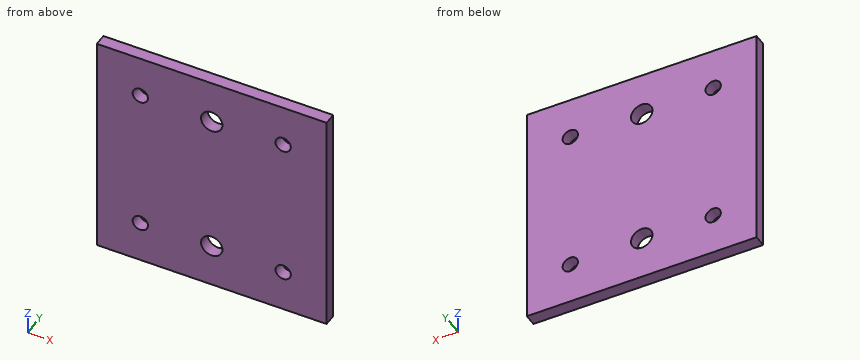
```python
from build123d import *

# Parameters (mm, degrees)
SKETCH1_W           = 150
SKETCH1_H           = 7.962213225
BOSS_EXTRUDE1_DEPTH = 150
SKETCH2_R           = 7
CUT_EXTRUDE1_DEPTH  = 8.962213225
SKETCH3_R           = 5
CUT_EXTRUDE2_DEPTH  = 8.962213225


with BuildPart() as part:
    # Sketch1 → Boss-Extrude1 (new body)
    with BuildSketch(Plane(origin=(0, 0, 0), x_dir=(0, 0, -1), z_dir=(1, 0, 0))):
        with Locations((75, -3.981106613)):
            Rectangle(SKETCH1_W, SKETCH1_H)
    extrude(amount=BOSS_EXTRUDE1_DEPTH)

    # Sketch2 → Cut-Extrude1 (cut, through all)
    with BuildSketch(Plane(origin=(0, 0, 0), x_dir=(1, 0, 0), z_dir=(0, 1, 0))):
        with Locations((74.999907539, 121.3473939)):
            Circle(SKETCH2_R)
        with Locations((74.999907539, 28.6526061)):
            Circle(SKETCH2_R)
    extrude(amount=-CUT_EXTRUDE1_DEPTH, mode=Mode.SUBTRACT)

    # Sketch3 → Cut-Extrude2 (cut, through all)
    with BuildSketch(Plane.XZ.offset(7.962213225)):
        with Locations((28.371496461, -122.5)):
            Circle(SKETCH3_R)
        with Locations((28.371496461, -27.5)):
            Circle(SKETCH3_R)
        with Locations((121.628503539, -27.5)):
            Circle(SKETCH3_R)
        with Locations((121.628503539, -122.5)):
            Circle(SKETCH3_R)
    extrude(amount=-CUT_EXTRUDE2_DEPTH, mode=Mode.SUBTRACT)


solid = part.part
```
Source: CAD feature listing. Evaluate the final solid. Frame: model axes, mm. Give positions to 0.01 mm unless a question says otherwise; leave off trailing zeros. Loops run counter-clockwise (first coordinate to the right, second up) from the corner with the lowest first, then second, coordinate; pieces in that order, holes last. Notation, with made-up numbers: (67.25, 60) -> (87.25, 60) arc R31 ccw to (87.25, 96) -> close; hole circle Ø9 at (78, 43). An arc over 180 degrees is marked (long way). Use a Markdown table: item, result. Add a question column.
(1) Section query B-B (y = -6.25). Output: boundary loops of the cut face in (x, z).
(2) Ray query, line 1 (X direction, y = -3.5, z = -25.5); line 2 (Z direction, x = 81, y = -7); line 3 (Z direction, x = 70.5, y = -3.75). Return the intervals inside material, ascending.
(3) First-contact query: pin 1 Ø9 at (x, z) = (121.63, -27.5) entering from +Y. Flat tip, straight axial feed; report the tip coordinate or a pass-through.
(4) Section query A-A (x = 70.5). Output: boundary loops of the cut face in (y, z).
Checked values:
| question | item | result |
|---|---|---|
| 1 | outline | (0, -150) -> (150, -150) -> (150, 0) -> (0, 0) -> close; hole circle Ø10 at (28.37, -122.5); hole circle Ø10 at (28.37, -27.5); hole circle Ø14 at (75, -121.35); hole circle Ø14 at (75, -28.65); hole circle Ø10 at (121.63, -122.5); hole circle Ø10 at (121.63, -27.5) |
| 2 | line 1 | 0 to 23.79, 32.95 to 68.75, 81.25 to 117.05, 126.21 to 150 |
| 2 | line 2 | -150 to -124.95, -117.74 to -32.26, -25.05 to 0 |
| 2 | line 3 | -150 to -126.71, -115.99 to -34.01, -23.29 to 0 |
| 3 | pin 1 | through |
| 4 | outline | (-7.96, -150) -> (0, -150) -> (0, -126.71) -> (-7.96, -126.71) -> close; (-7.96, -115.99) -> (0, -115.99) -> (0, -34.01) -> (-7.96, -34.01) -> close; (-7.96, -23.29) -> (0, -23.29) -> (0, 0) -> (-7.96, 0) -> close |
